Verification items for the finished model (mm, model axes). Face numbers are marked on the shaded views. A direction names the side the tool comes from. Round coordinates to 2 decimals unless told otherwise and drop trailing zeros. Loops run counter-clockwise (first coordinate to the right, second up) from the corner with the lowest first, then second, coordinate; pieces in that order, holes last. Notation, with made-up numbers: (3.25, -19) -> (34.25, -19) arc R19 ccw to (34.25, 12) -> close; hole circle Ø6 at (18.25, 58.25). An arc over 180 degrees is marked (long way). Use CSV: the item, a comma, the result in double quotes. Start each with the question number.
```python
from build123d import *

# Parameters (mm, degrees)
SKETCH1_R             = 7.5
BOSS_EXTRUDE1_DEPTH   = 3
CUT_EXTRUDE1_DEPTH    = 3
SKETCH6_W             = 1.811249569
SKETCH6_H             = 3.8
CUT_EXTRUDE2_DEPTH    = 3
F_2_0MM_DOWEL_HOLE1_D = 2


with BuildPart() as part:
    # Sketch1 → Boss-Extrude1 (new body)
    with BuildSketch(Plane.XY):
        Circle(SKETCH1_R)
    extrude(amount=BOSS_EXTRUDE1_DEPTH)

    # Sketch5 → Cut-Extrude1 (cut)
    with BuildSketch(Plane.XY.offset(3)):
        with BuildLine():
            Line((-1.811249569, 1.9), (-1.811249569, -1.9))
            ThreePointArc((-1.811249569, -1.9), (-2.625, 0), (-1.811249569, 1.9))
        make_face()
    cut_extrude1 = extrude(amount=-CUT_EXTRUDE1_DEPTH, mode=Mode.SUBTRACT)

    # Sketch6 → Cut-Extrude2 (cut)
    with BuildSketch(Plane.XY.offset(3)):
        with Locations((-0.905624785, 0)):
            Rectangle(SKETCH6_W, SKETCH6_H)
    cut_extrude2 = extrude(amount=-CUT_EXTRUDE2_DEPTH, mode=Mode.SUBTRACT)

    # Mirror1: Cut-Extrude1, Cut-Extrude2 across plane
    add(cut_extrude1.mirror(Plane(origin=(0, 0, 0), x_dir=(0, 0, 1), z_dir=(1, 0, 0))), mode=Mode.SUBTRACT)
    add(cut_extrude2.mirror(Plane(origin=(0, 0, 0), x_dir=(0, 0, 1), z_dir=(1, 0, 0))), mode=Mode.SUBTRACT)

    # Ø2.0mm Dowel Hole1 (through all)
    with Locations(Plane.XY.offset(3)):
        with Locations((5, 0), (-5, 0)):
            Hole(F_2_0MM_DOWEL_HOLE1_D / 2)


solid = part.part
```
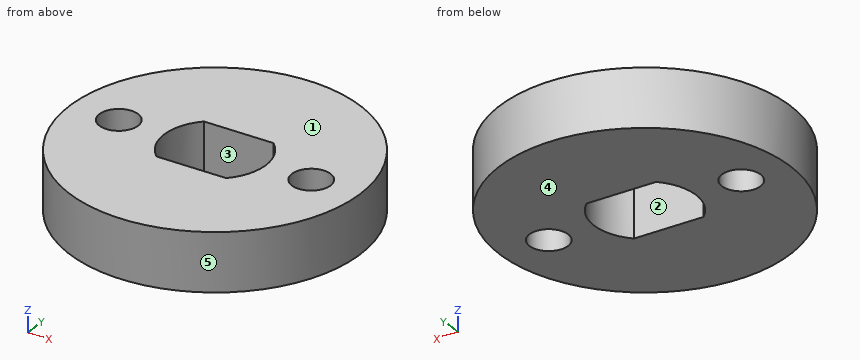
Q1. Cross-section at B-B (x = 0). Record the boundary of the cut face in (y, z), and give its area (3 significant figures).
Q2. Cross-section at D-D (x = -5.25). Record the boundary of the cut face in (y, z).
Q3. Depth check by flat-ended pin: pin 1 Ø1.8 at (x, y) = (5, 0) entering from -Z. Enter the tip coordinate at first touch or a pass-through.
Q4. Cross-section at A-A (y = 0). Record the boundary of the cut face in (x, z) (3 decimals), and give its area (4 significant figures).
Q5. Cross-section at C-C (z = 2.25). Record the boundary of the cut face in (x, y) (3 decimals).
Q6. Thickness scan on L1, parallel to Y at x = 0.25, z = 1.05; L2, parallel to Y at x = 1, z = 2.7; L3, parallel to X at y = -1.25, z = 2.7. Record the ranges inside material, lowest first. Write a range as from..to.
Q7. Release check for a two-part mould opening along Y. For the marked faces 3, 4 and 5 record: +Y half, -Y half, draft (parallel to the pull), parting line (faces both ways), or undercut.
Q8. Tool access check on the marked faces 1 and 2. Record the directions out of +Z, -Z, +X, -X, +Y, -Y that give a thin tool (end or side, any length) a straight path to the whole face; none if there is none.
Answer list:
1,outline,"(-7.5, 0) -> (-1.9, 0) -> (-1.9, 3) -> (-7.5, 3) -> close; (1.9, 0) -> (7.5, 0) -> (7.5, 3) -> (1.9, 3) -> close"
1,area,"33.6 mm2"
2,outline,"(-5.36, 0) -> (-0.97, 0) -> (-0.97, 3) -> (-5.36, 3) -> close; (0.97, 0) -> (5.36, 0) -> (5.36, 3) -> (0.97, 3) -> close"
3,pin 1,"passes through"
4,outline,"(-7.5, 0) -> (-6, 0) -> (-6, 3) -> (-7.5, 3) -> close; (-4, 0) -> (-2.625, 0) -> (-2.625, 3) -> (-4, 3) -> close; (2.625, 0) -> (4, 0) -> (4, 3) -> (2.625, 3) -> close; (6, 0) -> (7.5, 0) -> (7.5, 3) -> (6, 3) -> close"
4,area,"17.25 mm2"
5,outline,"circle Ø15 at (0, 0); hole circle Ø2 at (-5, 0); hole (-1.811, -1.9) -> (1.811, -1.9) arc R2.625 ccw to (1.811, 1.9) -> (-1.811, 1.9) arc R2.625 ccw to start; hole circle Ø2 at (5, 0)"
6,L1,"y = -7.5..-1.9, 1.9..7.5"
6,L2,"y = -7.43..-1.9, 1.9..7.43"
6,L3,"x = -7.4..-2.31, 2.31..7.4"
7,face 3,"undercut"
7,face 4,"draft"
7,face 5,"parting line"
8,face 1,"+Z, +X, -X, +Y, -Y"
8,face 2,"+Z, -Z"
